Geometry: see drawing. Coordinates: mm, zero at the bounding-box minimum. Give positions to 0.01 mm unless a question says otherwise; leave off trailing zeros. Order: outer loops, then holes, each group sorted by start corner. A loop starts at its lowest first (then second) coordinate and runs counter-clockwise, first axis right, second up. Notation, with made-up numbers: (40.5, 24) -> (86.5, 24) arc R17 ccw to (86.5, 41) -> close; hole circle Ø2 at (71.25, 28). An arc over 180 degrees is marked (long way). One line per item, written item: value. Start each with the question number.
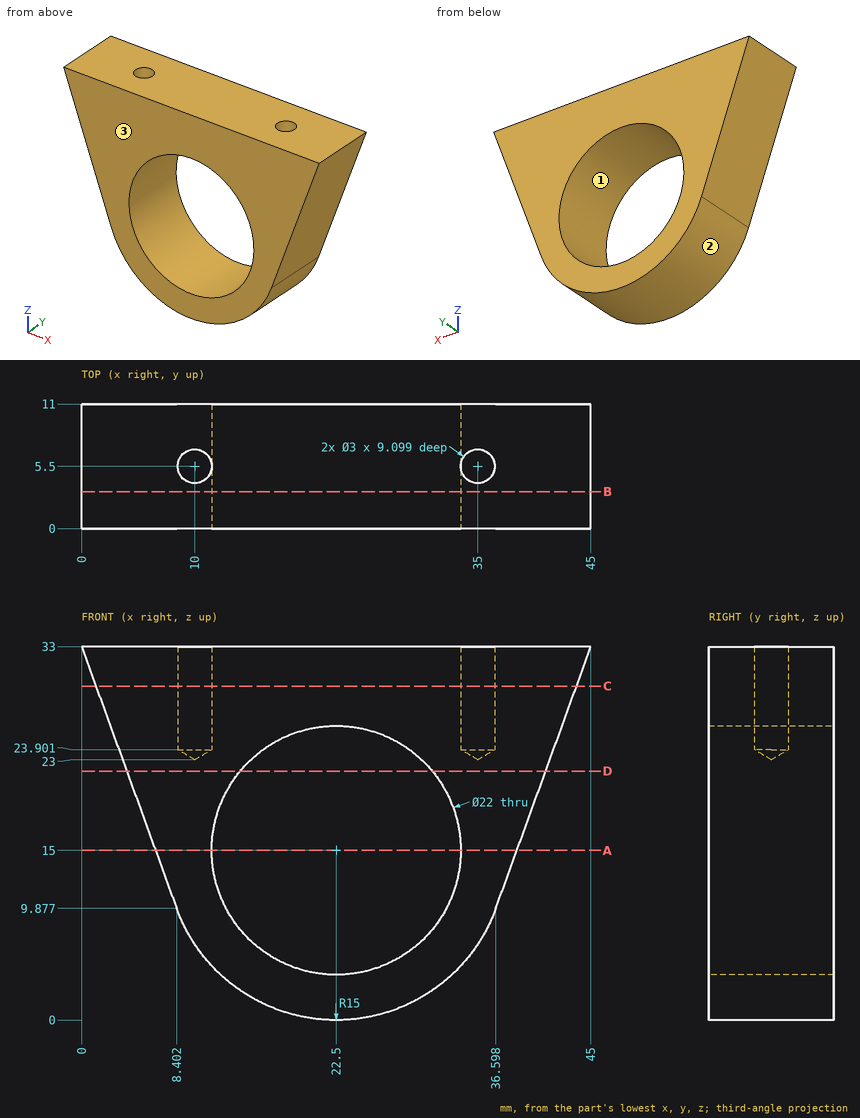
1. Material intervals for L1, parallel to Y at x = 35, z = 28; L2, parallel to X at y = 5.5, z = 27; L3, parallel to X at y = 5.5, z = 28, sorted ascending. Write a range as [from, to].
2. Pin query (flat end, axial travel): P1, Ø4, axis at y = 3.5, z = 8.5, coming from the +X side (1 decimal); P2, Ø12, axis at x = 6.5, z = 13.5, coming from the +Y side; P3, Ø17.5, axis at x = 22.5, z = 15, coming from the -Y side; P4, Ø2.5, axis at x = 35, y = 5.5, coming from the +Z side. Return the tip coordinate at first contact, or that it passes through.
3. Cut plane C-C, the plane z = 29.5. Return loops of the section in (x, y), then the cut area to 3 significant figures.
4. Cut plane A-A, the plane z = 15. Return loops of the section in (x, y).
5. Draft query along Z for the marked faces 1, 2 and 3. Return one class per face: pulls with the +Z half, pulls with the -Z half, needs draft (parallel to the pull), parting line crosses it, or undercut.
6. Cut plane D-D, the plane z = 22. Return loops of the section in (x, y) (1 decimal).
7. Cut plane B-B, the plane y = 3.25. Return loops of the section in (x, z), then the cut area to 3 significant figures.
Answers follow:
1. L1: y = [0, 4], [7, 11]
1. L2: x = [2.18, 8.5], [11.5, 33.5], [36.5, 42.82]
1. L3: x = [1.82, 8.5], [11.5, 33.5], [36.5, 43.18]
2. P1: stops at x = 36.8
2. P2: stops at y = 11
2. P3: passes through
2. P4: stops at z = 23.75
3. outline: (1.27, 0) -> (43.73, 0) -> (43.73, 11) -> (1.27, 11) -> close; hole circle Ø3 at (10, 5.5); hole circle Ø3 at (35, 5.5)
3. area: 453 mm²
4. outline: (6.54, 0) -> (11.5, 0) -> (11.5, 11) -> (6.54, 11) -> close; (33.5, 0) -> (38.46, 0) -> (38.46, 11) -> (33.5, 11) -> close
5. face 1: undercut
5. face 2: pulls with the -Z half
5. face 3: needs draft
6. outline: (4, 0) -> (14, 0) -> (14, 11) -> (4, 11) -> close; (31, 0) -> (41, 0) -> (41, 11) -> (31, 11) -> close
7. outline: (0, 33) -> (8.4, 9.88) arc R15 ccw to (36.6, 9.88) -> (45, 33) -> close; hole circle Ø22 at (22.5, 15)
7. area: 669 mm²
